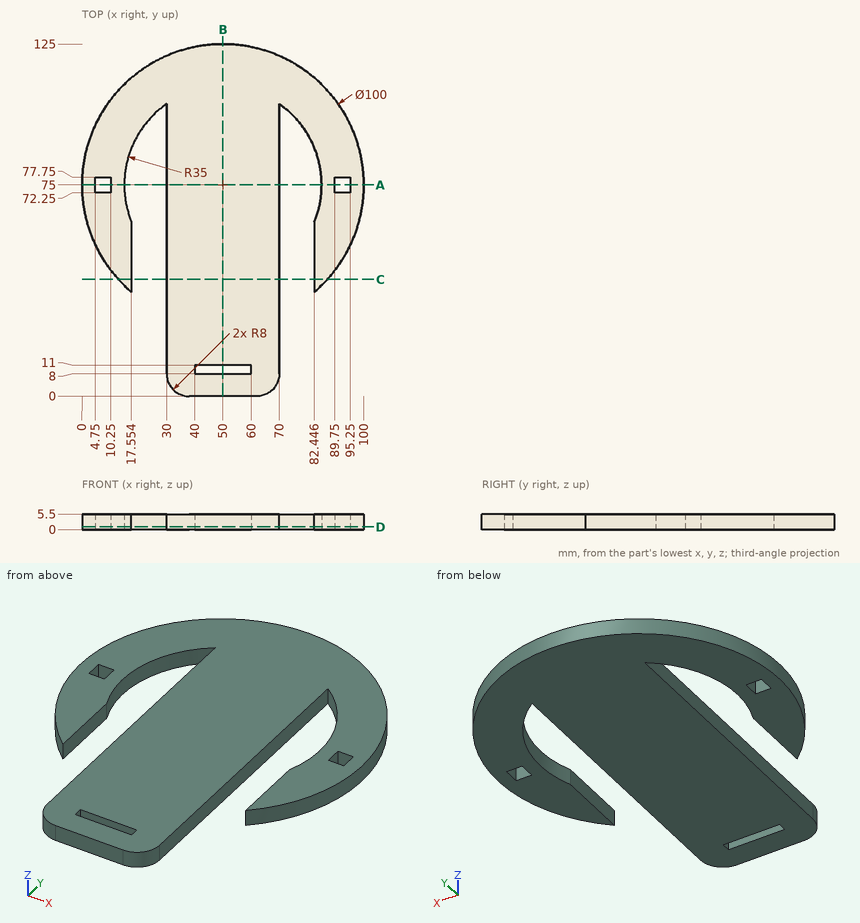
Print and shaded views of the part. All mm, measured from the part's lowest x, y and z. Coordinates: 2 decimals unless noted, no trailing zeros. Order: outer loops, then holes, each group sorted by start corner. A loop starts at its lowest first (then second) coordinate and runs counter-clockwise, first axis right, second up. Notation, with made-up numbers: (23, 15) - (28, 15) arc R11 ccw to (28, 31) - close; hole circle Ø7 at (-7, 79.5). An arc over 180 degrees is marked (long way). Put each result on its own line as item: value.
1. Drop flat-ended pins along their axis: P1, Ø1.6, axis at x = 46, z = 2, coming from the +Y side; P2, Ø1.6, axis at y = 43.5, z = 3, coming from the -X side (1 decimal); P3, Ø1, axis at x = 81, z = 4.5, coming from the +Y side. Give the stop position or say it passes through.
Answer sheet:
P1: stops at y = 124.9
P2: stops at x = 10.5
P3: stops at y = 114.62
2. Probe line 1 along X through (y, z) = (56, 2.9); line 2 along X through (y, z) = (50.5, 3.2); line 3 along Y through (x, z) = (10, 1.45). List the from-to ranges inside material, lowest first. Write a range as [from, to].
Answer sheet:
line 1: x = [3.75, 17.55], [30, 70], [82.45, 96.25]
line 2: x = [6.41, 17.55], [30, 70], [82.45, 93.59]
line 3: y = [45, 72.25], [77.75, 105]
3. Saw through at B-B (x = 50). Write the cut outline in (y, z).
Answer sheet:
outline: (0, 0) - (8, 0) - (8, 5.5) - (0, 5.5) - close; (11, 0) - (125, 0) - (125, 5.5) - (11, 5.5) - close
4. Saw through at D-D (z = 1). Write the cut outline in (x, y) (3 decimals), and give its area (3 significant figures).
Answer sheet:
outline: (17.554, 36.957) - (17.554, 61.875) arc R35 cw to (30, 103.723) - (30, 8) arc R8 ccw to (38, 0) - (62, 0) arc R8 ccw to (70, 8) - (70, 103.723) arc R35 cw to (82.446, 61.875) - (82.446, 36.957) arc R50 ccw (long way) to start; hole (4.75, 72.25) - (10.25, 72.25) - (10.25, 77.75) - (4.75, 77.75) - close; hole (40, 8) - (60, 8) - (60, 11) - (40, 11) - close; hole (89.75, 72.25) - (95.25, 72.25) - (95.25, 77.75) - (89.75, 77.75) - close
area: 7,060 mm^2
5. Saw through at C-C (y = 41.5). Write the cut outline in (x, z), and give its area (3 significant figures).
Answer sheet:
outline: (12.88, 0) - (17.55, 0) - (17.55, 5.5) - (12.88, 5.5) - close; (30, 0) - (70, 0) - (70, 5.5) - (30, 5.5) - close; (82.45, 0) - (87.12, 0) - (87.12, 5.5) - (82.45, 5.5) - close
area: 271 mm^2
6. Saw through at A-A (y = 75). Write the cut outline in (x, z), and give its area (4 significant figures).
Answer sheet:
outline: (0, 0) - (4.75, 0) - (4.75, 5.5) - (0, 5.5) - close; (10.25, 0) - (15, 0) - (15, 5.5) - (10.25, 5.5) - close; (30, 0) - (70, 0) - (70, 5.5) - (30, 5.5) - close; (85, 0) - (89.75, 0) - (89.75, 5.5) - (85, 5.5) - close; (95.25, 0) - (100, 0) - (100, 5.5) - (95.25, 5.5) - close
area: 324.5 mm^2
